Could you check a few things on this model? Use its own coordinates, in mm. Face numbers are marked on the shaded views. A direction names the side the tool comes from. Give positions to 0.01 mm unless a question says otherwise; leave off trailing zeros. Loops run counter-clockwise (first coordinate to the right, second up) from the corner with the lowest first, then second, coordinate; pieces in that order, holes last. Notation, with made-up numbers: (47.25, 53.5) -> (100.25, 53.5) arc R7 ccw to (100.25, 60.5) -> close; hole circle Ø5 at (38, 65.5). An arc over 180 degrees is marked (long way). Write item = value, one per line. Start each with the question number.
1) I'm going to push flat-ended pins straight in: pin 1 Ø1.5 at (x, y) = (-0.5, 5) entering from +Z; pin 2 Ø1.5 at (x, y) = (1.5, 13) entering from -Z; pin 3 Ø3 at (x, z) = (1.5, 2.5) entering from +Y. Where does each tip first touch, or does it pass through?
2) I want a section at A-A (y = 7.5). List the corners of the cut face in (x, z) for me (3 decimals).
3) If we mould it in two halves opening along X, with no side actions, what happens to the marked faces 3, 4, 5 and 6? For each: +X half, -X half, draft (parallel to the pull), parting line (faces both ways), or undercut.
4) I want a section at C-C (z = -2.3). List the corners of the cut face in (x, y) for me, and give its area (3 significant figures).
5) I need wall thicknesses on probe 1 along X at (y, z) = (6.75, 0) (3 decimals); probe 2 along Y at (x, z) = (1.35, 1.5); probe 3 along X at (y, z) = (7.25, 0.4). Which ranges of each line are inside material? Lowest first, please. Write a range as from..to.
6) On a 3-axis mill with a long thin cutter (end or side, diameter ignored), from which of +Z, -Z, +X, -X, +Y, -Y can I reach the whole of each face in a straight line? I mean the marked faces 1 and 2. Say none if no direction works.
7) I want a section at B-B (y = 13.75). List the corners of the cut face in (x, z) for me, and give its area (3 significant figures).
8) I want a section at D-D (x = -2.2). List the corners of the cut face in (y, z) for me, and give its area (3 significant figures).
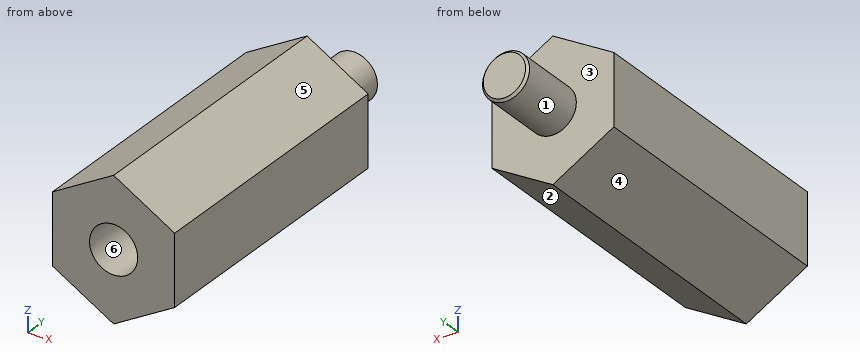
from build123d import *

# Parameters (mm, degrees)
EXTRUDE_1_DEPTH  = 12
SKETCH_2_R       = 1
EXTRUDE_2_DEPTH  = 3
M2_5X0_451_D     = 2.05
M2_5X0_451_DEPTH = 10
M2_5X0_451_TIP   = 0.615882135
CHAMFER_1_SIZE   = 0.1


with BuildPart() as part:
    # Эскиз1 → Бобышка-Вытянуть1 (new body)
    with BuildSketch(Plane(origin=(0, 0, 0), x_dir=(1, 0, 0), z_dir=(0, 1, 0))):
        Polygon((0, 3), (-2.598076211, 1.5), (-2.598076211, -1.5), (0, -3), (2.598076211, -1.5), (2.598076211, 1.5), align=None)
    extrude(amount=EXTRUDE_1_DEPTH)

    # Эскиз2 → Бобышка-Вытянуть2 (add)
    with BuildSketch(Plane(origin=(0, 12, 0), x_dir=(1, 0, 0), z_dir=(0, 1, 0))):
        with Locations(Location((0, 0, 0), (0, 0, 270))):
            Circle(SKETCH_2_R)
    extrude(amount=EXTRUDE_2_DEPTH)

    # Отверстие обработанное метчиком M2.5x0.451
    with Locations(Plane(origin=(0, 0, 0), x_dir=(0, 0, -1), z_dir=(0, -1, 0))):
        with Locations((0, 0)):
            Hole(M2_5X0_451_D / 2, depth=M2_5X0_451_DEPTH)
            with Locations((0, 0, -(M2_5X0_451_DEPTH + M2_5X0_451_TIP / 2))):  # 118° drill point
                Cone(0, M2_5X0_451_D / 2, M2_5X0_451_TIP, mode=Mode.SUBTRACT)

    # Фаска1
    chamfer_1_edges = [part.edges().sort_by_distance(p)[0] for p in [
        (0, 15, -1),
    ]]
    chamfer(chamfer_1_edges, length=CHAMFER_1_SIZE)


solid = part.part
Answer list:
q1.pin_1 = 3
q1.pin_2 = -0.66
q1.pin_3 = 12
q2.outline = (-2.598, -1.5) -> (0, -3) -> (2.598, -1.5) -> (2.598, 1.5) -> (0, 3) -> (-2.598, 1.5) -> close; hole circle Ø2.05 at (0, 0)
q3.face_3 = draft
q3.face_4 = -X half
q3.face_5 = +X half
q3.face_6 = undercut
q4.outline = (-1.21, 0) -> (1.21, 0) -> (1.21, 12) -> (-1.21, 12) -> close
q4.area = 29.1 mm^2
q5.probe_1 = -2.598..-1.025, 1.025..2.598
q5.probe_2 = 0..12
q5.probe_3 = -2.6..-0.94, 0.94..2.6
q6.face_1 = +Y
q6.face_2 = -Z, +X, +Y, -Y
q7.outline = circle Ø2 at (0, 0)
q7.area = 3.14 mm^2
q8.outline = (0, -1.73) -> (12, -1.73) -> (12, 1.73) -> (0, 1.73) -> close
q8.area = 41.5 mm^2
